Autodesk Inventor part; units mm, degrees
ref_plane "YZ Plane" through (0, 0, 0) normal (1, 0, 0) x (0, 1, 0)
ref_plane "XZ Plane" through (0, 0, 0) normal (0, 1, 0) x (-1, 0, 0)
ref_plane "XY Plane" through (0, 0, 0) normal (0, 0, 1) x (1, 0, 0)
sketch "Sketch1" plane through (0, 0, 0) normal (0, 0, 1) x (1, 0, 0)
  line L0 (0, 0) -> (3, 0)
  line L1 (3, 0) -> (3, 5)
  line L2 (3, 5) -> (1.4, 5)
  line L3 (1.4, 5) -> (1.4, 7.1)
  line L4 (1.4, 7.1) -> (3.5, 7.1)
  line L5 (3.5, 7.1) -> (3.5, 17.1)
  line L6 (3.5, 17.1) -> (3, 17.1)
  line L7 (3, 17.1) -> (3, 21.2)
  line L8 (3, 21.2) -> (0, 21.2)
  line L9 (0, 21.2) -> (0, 0)
  dimension "d0" = 2.1
  dimension "d1" = 7.1
  dimension "d3" = 10
  dimension "d4" = 14.1
  dimension "d5" = 3
  dimension "d6" = 1.4
  dimension "d7" = 3.5
  dimension "d8" = 3
revolve "Revolution1" add sketch "Sketch1" angle 360 about axis through (0, 21.2, 0) along (0, -1, 0)
thread "Thread1"
thread "Thread2"
sketch "Sketch2" plane through (0, 21.2, 0) normal (0, 1, 0) x (1, 0, 0)
  circle A0 centre (0, 0) radius 3
  point P0 (0, 0)
hole "Hole1" at (0, 21.2, 0) direction (0, -1, 0) diameter 2 end through all
hole "Hole2" at (0, 21.2, 0) direction (0, -1, 0) diameter 4.2 depth 5 tip angle 118
chamfer "Chamfer1" distance 0.25 angle 45 1 edges at (-3, 21.2, 0)
chamfer "Chamfer2" distance 0.25 angle 45 1 edges at (-3, 0, 0)
properties part number "Heatbreak" material "Stainless Steel"
Can you work these out from the model? Positions are in its coordinate system, mm. A direction names the side the tool comes from. Coordinates: 2 decimals unless noted, no trailing zeros. Write each loop counter-clockwise with the first axis right and the second up, starting at its lowest first coordinate (ties: lowest second). Pieces come first, ordered by that corner, then holes. Notation, with made-up numbers: (49.5, 19.25) -> (99.5, 19.25) arc R18 cw to (99.5, 51.25) -> close; hole circle Ø2 at (42, 1.25). An arc over 180 degrees is marked (long way). Write each question's results on one line, items separated by ' | '. Start each with the question number.
Q1. Imagine slicing it at C-C (y = 17.75). Write out the boundary of the cut face in (x, z), then the cut area to 3 significant figures.
Q2. On a 3-axis mill with a long thin cutter (end or side, diameter ignored), from which of +Z, -Z, +X, -X, +Y, -Y can I reach the whole of each face in a straight line? I mean faces 4 (the face through (-3, 19, 0)), 5 (the face through (-3, 3, 0)), 6 (the face through (-1.4, 6.06, -0.06)). Say none if no direction works.
Q3. If I drill on probe 1 along Y at (x, z) = (1.75, -1.5); probe 2 along Z at (x, y) = (0, 19.5); probe 3 along Y at (x, z) = (-2.75, -1.75), over which ranges is the centre line in solid material (lowest first)?
Q4. Imagine slicing it at D-D (y = 3.75). Write out the boundary of the cut face in (x, z).
Q5. I'm going to push flat-ended pins straight in: pin 1 (1 mm diameter, centred on x = 2.5, y = 10.5, fed in from +Z); pin 2 (2 mm diameter, centred on y = 19, z = -2.5, fed in from +X); pin 3 (1 mm diameter, centred on x = 0.5, y = 6, fed in from +Z). Where does each tip first touch, or does it pass through?
Q6. Imagine slicing it at A-A (z = 0). Write out the boundary of the cut face in (x, y), then the cut area to 3 significant figures.
Q7. Imagine slicing it at B-B (x = 0). Write out the boundary of the cut face in (y, z), then the cut area to 3 significant figures.
Q8. We'd pull the mould along X, two halves only. Please class faces 1 (the face through (-0.631, 18.665, 2.003)), 2 (the face through (3, 17.1, 1)), 3 (the face through (3.233, 12.17, 1.341)): +X half, -X half, draft (parallel to the pull), parting line (faces both ways), or undercut.
Taken from the geometry:
1) outline: circle Ø6 at (0, 0); hole circle Ø4.2 at (0, 0) | area: 14.4 mm^2
2) face 4: +Y | face 5: -Y | face 6: none
3) probe 1: y = 0 to 5, 7.1 to 21.2 | probe 2: z = -3 to -2.1, 2.1 to 3 | probe 3: y = 7.1 to 17.1
4) outline: circle Ø6 at (0, 0); hole circle Ø2 at (0, 0)
5) pin 1: stops at z = 2.87 | pin 2: stops at x = 2.6 | pin 3: stops at z = 1.4
6) outline: (-3.5, 7.1) -> (-1.4, 7.1) -> (-1.4, 5) -> (-3, 5) -> (-3, 0.25) -> (-2.75, 0) -> (-1, 0) -> (-1, 15.54) -> (-2.1, 16.2) -> (-2.1, 21.2) -> (-2.75, 21.2) -> (-3, 20.95) -> (-3, 17.1) -> (-3.5, 17.1) -> close; (1, 0) -> (2.75, 0) -> (3, 0.25) -> (3, 5) -> (1.4, 5) -> (1.4, 7.1) -> (3.5, 7.1) -> (3.5, 17.1) -> (3, 17.1) -> (3, 20.95) -> (2.75, 21.2) -> (2.1, 21.2) -> (2.1, 16.2) -> (1, 15.54) -> close | area: 76.2 mm^2
7) outline: (0, -2.75) -> (0.25, -3) -> (5, -3) -> (5, -1.4) -> (7.1, -1.4) -> (7.1, -3.5) -> (17.1, -3.5) -> (17.1, -3) -> (20.95, -3) -> (21.2, -2.75) -> (21.2, -2.1) -> (16.2, -2.1) -> (15.54, -1) -> (0, -1) -> close; (0, 1) -> (15.54, 1) -> (16.2, 2.1) -> (21.2, 2.1) -> (21.2, 2.75) -> (20.95, 3) -> (17.1, 3) -> (17.1, 3.5) -> (7.1, 3.5) -> (7.1, 1.4) -> (5, 1.4) -> (5, 3) -> (0.25, 3) -> (0, 2.75) -> close | area: 76.2 mm^2
8) face 1: undercut | face 2: draft | face 3: parting line
